Autodesk Inventor part; units mm, degrees
ref_plane "YZ Plane" through (0, 0, 0) normal (1, 0, 0) x (0, 1, 0)
ref_plane "XZ Plane" through (0, 0, 0) normal (0, 1, 0) x (-1, 0, 0)
ref_plane "XY Plane" through (0, 0, 0) normal (0, 0, 1) x (1, 0, 0)
sketch "Sketch1" plane through (0, 0, 0) normal (1, 0, 0) x (0, 1, 0)
  line L0 (0, 0) -> (25.4, 0)
  line L1 (25.4, 0) -> (25.4, -25.4)
  line L2 (25.4, -25.4) -> (0, -25.4)
  line L3 (0, -25.4) -> (0, 0)
  line L4 (22.225, -3.175) -> (3.175, -3.175)
  line L5 (3.175, -3.175) -> (3.175, -22.225)
  line L6 (3.175, -22.225) -> (22.225, -22.225)
  line L7 (22.225, -22.225) -> (22.225, -3.175)
  dimension "d0" = 25.4
  dimension "d1" = 25.4
  dimension "d2" = 3.175
extrude "Extrusion1" add sketch "Sketch1" along normal blind 304.8
sketch "Sketch2" plane through (0, 0, 0) normal (0, 0, 1) x (1, 0, 0)
  circle A0 centre (273.05, 12.7) radius 23.8125 construction
  line L0 (0, 25.4) -> (304.8, 25.4) construction
  line L1 (304.8, 25.4) -> (304.8, 0) construction
  circle A1 centre (296.8625, 12.7) radius 2.54
  circle A2 centre (249.2375, 12.7) radius 2.54
  line L2 (304.8, 12.7) -> (0, 12.7) construction
  line L3 (0, 0) -> (0, 25.4) construction
  line L4 (276.7162, 19.05) -> (280.3823, 12.7) construction
  line L5 (280.3823, 12.7) -> (276.7162, 6.35) construction
  line L6 (276.7162, 6.35) -> (269.3838, 6.35) construction
  line L7 (269.3838, 6.35) -> (265.7177, 12.7) construction
  line L8 (265.7177, 12.7) -> (269.3838, 19.05) construction
  line L9 (269.3838, 19.05) -> (276.7162, 19.05) construction
  circle A3 centre (273.05, 12.7) radius 7.3323
  circle A4 centre (12.7, 12.7) radius 3.175
  circle A5 centre (38.1, 12.7) radius 3.175
  dimension "d5" = 47.625
  dimension "d6" = 12.7
  dimension "d7" = 31.75
  dimension "d8" = 5.08
  dimension "d9" = 5.08
  dimension "d10" = 12.7
  dimension "d13" = 6.35
  dimension "d14" = 6.35
  dimension "d15" = 12.7
  dimension "d16" = 25.4
extrude "Extrusion2" cut sketch "Sketch2" against normal blind 25.4
properties part number "1x1x12" material "Aluminum 6061"
Source: CAD feature listing. Evaluate the final solid. Frame: model axes, mm. A direction names the side the tool comes from. Give positions to 0.01 mm unless a question says otherwise; leave off trailing zeros. Write each loop counter-clockwise with the first axis right and the second up, starting at its lowest first coordinate (ties: lowest second). Pieces come first, ordered by that corner, then holes. Notation, with made-up numbers: (66.25, 57.25) -> (81.25, 57.25) arc R21 cw to (81.25, 94.25) -> close; hole circle Ø8 at (60, -25.5). An arc over 180 degrees is marked (long way). Return JSON: item names as keys, results as strings. Group by question number.
1. Section D-D, the plane x = 12.7. Output: boundary loops of the cut face in (y, z) (3 decimals).
2. Mould query, pull axis Y, two halves, no side actions, for faces 3 (the face through (298.23, 14.84, -23.79)), 4 (the face through (150, 13, 0)), 5 (the face through (150, 0, -13)). Classes: +Y half, -Y half, draft (parallel to the pull), parting line (faces both ways), or undercut.
3. Access query for faces 1 (the face through (150, 22.225, -13)), 2 (the face through (0, 24, -13)). Directions: +Z, -Z, +X, -X, +Y, -Y. A direction counts if a zero-diameter tool reaches every point of the face in a straight line with its end or side. Return the directions, or none.
4. Section B-B, the plane x = 149. Output: boundary loops of the cut face in (y, z) (3 decimals).
5. Material intervals for line 1 (Z direction, x = 155.5, y = 20) (3 decimals); line 2 (Y direction, x = 38.1, z = -23.55) (3 decimals); line 3 (Y direction, x = 157, z = -9.75) (3 decimals), sorted ascending. Write a range as from..to.
6. Section A-A, the plane x = 273.05. Output: boundary loops of the cut face in (y, z) (3 decimals), then the cut area to 3 significant figures.
7. Pin query (flat end, axial travel): pin 1 Ø9 at (x, y) = (273.05, 12.7) entering from +Z. Return the tip coordinate at first contact, or that it passes through.
8. Section C-C, the plane y = 12.7. Count the separate pieces of the cut face and the enclosed holes in it, then the cut area to 3 significant figures.
Determined:
{
 "1": {"outline": "(0, -25.4) -> (9.525, -25.4) -> (9.525, -22.225) -> (3.175, -22.225) -> (3.175, -3.175) -> (9.525, -3.175) -> (9.525, 0) -> (0, 0) -> close; (15.875, -25.4) -> (25.4, -25.4) -> (25.4, 0) -> (15.875, 0) -> (15.875, -3.175) -> (22.225, -3.175) -> (22.225, -22.225) -> (15.875, -22.225) -> close"},
 "2": {"face 3": "undercut", "face 4": "draft", "face 5": "-Y half"},
 "3": {"face 1": "+X, -X", "face 2": "+Z, -Z, -X, +Y, -Y"},
 "4": {"outline": "(0, -25.4) -> (25.4, -25.4) -> (25.4, 0) -> (0, 0) -> close; hole (3.175, -22.225) -> (22.225, -22.225) -> (22.225, -3.175) -> (3.175, -3.175) -> close"},
 "5": {"line 1": "z = -25.4..-22.225, -3.175..0", "line 2": "y = 0..9.525, 15.875..25.4", "line 3": "y = 0..3.175, 22.225..25.4"},
 "6": {"outline": "(0, -25.4) -> (5.368, -25.4) -> (5.368, -22.225) -> (3.175, -22.225) -> (3.175, -3.175) -> (5.368, -3.175) -> (5.368, 0) -> (0, 0) -> close; (20.032, -25.4) -> (25.4, -25.4) -> (25.4, 0) -> (20.032, 0) -> (20.032, -3.175) -> (22.225, -3.175) -> (22.225, -22.225) -> (20.032, -22.225) -> close", "area": "189 mm2"},
 "7": {"pin 1": "passes through"},
 "8": {"separate pieces": "12", "enclosed holes": "0", "area": "1,700 mm2"}
}
